CAD build for the part. Positions are in the model's coordinates, mm. A direction names the side the tool comes from. Round coordinates to 2 decimals unless told otherwise and drop trailing zeros. Write each loop counter-clockwise with the first axis right and the second up, starting at its lowest first coordinate (ties: lowest second). Pieces come first, ordered by that corner, then holes. Notation, with made-up numbers: (45, -38.5) - (90, -38.5) arc R29 ccw to (90, -10.5) - close; hole circle Ø3 at (59, 19.5). An arc over 180 degrees is marked (long way). Put each result on its own line as item: value. Start each with the question number.
Item 1: 3-axis set-ups, long thin cutter, end or side, ignore diameter. For faces 4 (the flat face through (0, 6, 640)), 5 (the cylindrical face through (13.347, 34.812, 634.558)), 6 (the flat face through (15, 6.35, 635)): which of +Z, -Z, +X, -X, +Y, -Y reach the whole face in a straight line?
Item 2: Cut at A-A (x = 15). Give the cut face in (y, z), and give its area (3 significant figures).
Item 3: Drill centre lines: line 1 (Z direction, x = 27.5, y = 10.5); line 2 (Y direction, x = 17, z = 406); line 3 (Y direction, x = 5, z = 421.5). Where is each one in solid material? Low to high. Write a range as from..to.
Item 4: Cut at B-B (z = 458.5). Give the cut face in (x, y).
Item 5: Cut at C-C (y = 22.22). Give the cut face in (x, z), and give its area (3 significant figures).
Item 6: Mould opens along Y. For faces 1 (the flat face through (15, 0, 634)), 2 (the flat face through (15, 20, 1286)), 3 (the flat face through (18, 35, 1246)) say: released by +Y, released by -Y, zero draft, split by the parting line, or undercut.
Item 7: Pin check, flat tips, straight feed: pin 1 Ø3 at (x, z) = (23.5, 342) entering from +Y; pin 2 Ø15 at (x, z) = (22, 693.5) entering from +Y; pin 3 Ø12 at (x, y) = (6, 35.5) entering from -Z; pin 4 Ø4 at (y, z) = (16, 177) entering from +X. Stop position of each tip, or through.
```python
from build123d import *

# Parameters (mm, degrees)
SKETCH1_W           = 30
SKETCH1_H           = 40
BOSS_EXTRUDE1_DEPTH = 40
FILLET1_R           = 10.16
FILLET2_R           = 2.54
SKETCH3_R           = 12.7
BOSS_EXTRUDE2_DEPTH = 1206
SKETCH6_W           = 30
SKETCH6_H           = 40
BOSS_EXTRUDE3_DEPTH = 40.00000001
FILLET3_R           = 10.16
FILLET4_R           = 2.54
SKETCH7_W           = 30
SKETCH7_H           = 6.35
BOSS_EXTRUDE4_DEPTH = 1206
FILLET5_R           = 2.54


with BuildPart() as part:
    # Sketch1 → Boss-Extrude1 (new body)
    with BuildSketch(Plane.XY):
        with Locations((15, 20)):
            Rectangle(SKETCH1_W, SKETCH1_H)
    extrude(amount=BOSS_EXTRUDE1_DEPTH)

    # Fillet1
    fillet1_edges = [part.edges().sort_by_distance(p)[0] for p in [
        (0, 40, 20),
        (30, 40, 20),
    ]]
    fillet(fillet1_edges, radius=FILLET1_R)

    # Fillet2
    fillet2_edges = [part.edges().sort_by_distance(p)[0] for p in [
        (30, 0, 20),
        (0, 0, 20),
    ]]
    fillet(fillet2_edges, radius=FILLET2_R)

    # Sketch3 → Boss-Extrude2 (add)
    with BuildSketch(Plane.XY.offset(40)):
        with Locations((15, 22.22)):
            Circle(SKETCH3_R)
    extrude(amount=BOSS_EXTRUDE2_DEPTH)

    # Sketch6 → Boss-Extrude3 (add)
    with BuildSketch(Plane.XY.offset(1246)):
        with Locations((15, 20)):
            Rectangle(SKETCH6_W, SKETCH6_H)
    extrude(amount=BOSS_EXTRUDE3_DEPTH)

    # Fillet3
    fillet3_edges = [part.edges().sort_by_distance(p)[0] for p in [
        (0, 40, 1266.000000005),
        (30, 40, 1266.000000005),
    ]]
    fillet(fillet3_edges, radius=FILLET3_R)

    # Fillet4
    fillet4_edges = [part.edges().sort_by_distance(p)[0] for p in [
        (0, 0, 1266.000000005),
        (30, 0, 1266.000000005),
    ]]
    fillet(fillet4_edges, radius=FILLET4_R)

    # Sketch7 → Boss-Extrude4 (add)
    with BuildSketch(Plane.XY.offset(40)):
        with Locations((15, 3.175)):
            Rectangle(SKETCH7_W, SKETCH7_H)
    extrude(amount=BOSS_EXTRUDE4_DEPTH)

    # Fillet5
    fillet5_edges = [part.edges().sort_by_distance(p)[0] for p in [
        (30, 0, 643),
        (0, 0, 643),
    ]]
    fillet(fillet5_edges, radius=FILLET5_R)


solid = part.part
```
Output values:
1. face 4: +Z, -Z, -X, +Y, -Y
1. face 5: none
1. face 6: +X, -X
2. outline: (0, 0) - (40, 0) - (40, 40) - (34.92, 40) - (34.92, 1246) - (40, 1246) - (40, 1286) - (0, 1286) - close; hole (6.35, 40) - (9.52, 40) - (9.52, 1246) - (6.35, 1246) - close
2. area: 41,500 mm2
3. line 1: 0..40, 1246..1286
3. line 2: 0..6.35, 9.68..34.76
3. line 3: 0..6.35, 14.39..30.05
4. outline: (0, 2.54) arc R2.54 ccw to (2.54, 0) - (27.46, 0) arc R2.54 ccw to (30, 2.54) - (30, 6.35) - (0, 6.35) - close; circle Ø25.4 at (15, 22.22)
5. outline: (0, 0) - (30, 0) - (30, 40) - (27.7, 40) - (27.7, 1246) - (30, 1246) - (30, 1286) - (0, 1286) - (0, 1246) - (2.3, 1246) - (2.3, 40) - (0, 40) - close
5. area: 33,000 mm2
6. face 1: released by -Y
6. face 2: zero draft
6. face 3: undercut
7. pin 1: y = 32.82
7. pin 2: y = 34.92
7. pin 3: z = 0
7. pin 4: x = 26.98
